Design review of the part shown in the three views and the two pictorial views. Dimensions are in mm from the part's minimum x, y and z. Coordinates: 2 decimals unless noted, no trailing zeros. Write each loop counter-clockwise with the first axis right and the second up, starting at its lowest first coordinate (ties: lowest second). Pieces come first, ordered by that corner, then holes.
Q1. Take a section at A-A, the plane y = 1.55. State how many separate pieces and enclosed holes the cut face has, plus the area to 3 significant figures.
Q2. For pin 1 Ø6.5 at (x, z) = (73.025, 6.35) entering from +Y, flat-tipped, find the tip position at first contact; note if it passes through.
Q3. Take a section at B-B, the plane z = 41. Write out the cut boundary in (x, y) (1 decimal).
Q4. For L1, parallel to Z at x = 6.5, y = 1.65; L2, parallel to Z at x = 70, y = 2.45; L3, parallel to Z at x = 73.5, y = 2.7, list the stretches that pass through material, from the lowest coordinate up.
Q5. Take a section at C-C, the plane x = 24. Write out the cut boundary in (y, z) (1 decimal), plus the area to 3 significant figures.
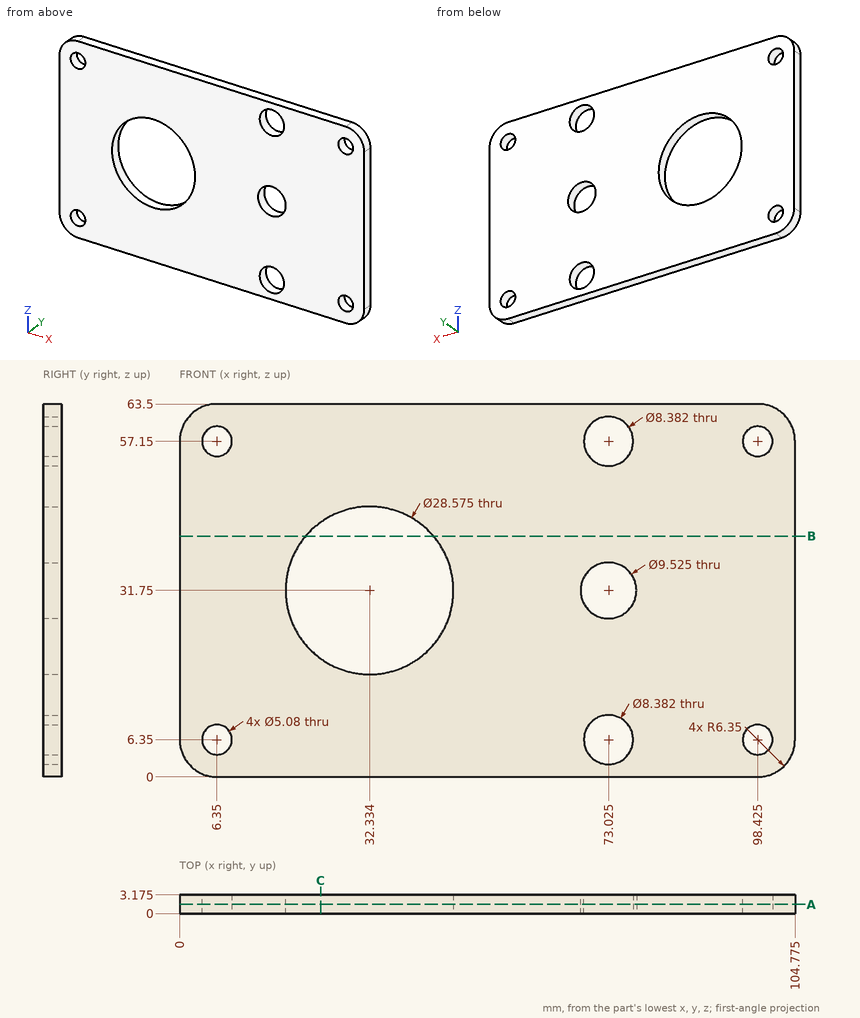
Responses:
1. separate pieces: 1
1. enclosed holes: 8
1. area: 5,710 mm2
2. pin 1: passes through
3. outline: (0, 0) - (21.4, 0) - (21.4, 3.2) - (0, 3.2) - close; (43.2, 0) - (104.8, 0) - (104.8, 3.2) - (43.2, 3.2) - close
4. L1: z = 0 to 3.81, 8.89 to 54.61, 59.69 to 63.5
4. L2: z = 0 to 3.45, 9.25 to 28.07, 35.43 to 54.25, 60.05 to 63.5
4. L3: z = 0 to 2.19, 10.51 to 27.01, 36.49 to 52.99, 61.31 to 63.5
5. outline: (0, 0) - (3.2, 0) - (3.2, 20.1) - (0, 20.1) - close; (0, 43.4) - (3.2, 43.4) - (3.2, 63.5) - (0, 63.5) - close
5. area: 128 mm2
